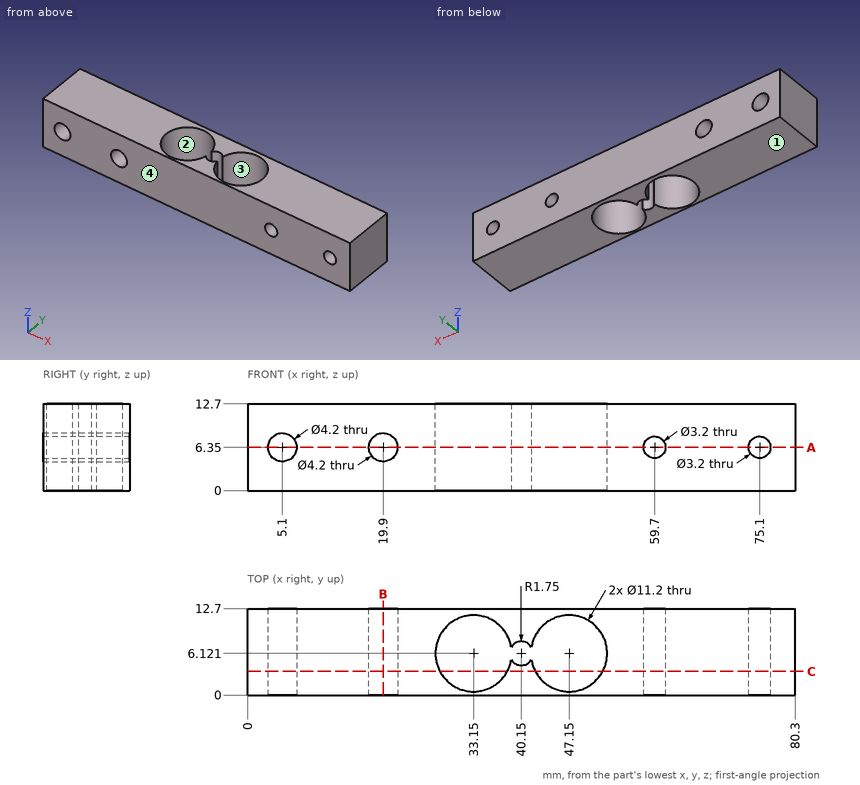
Study the drawing (mm; zero at the part's minimum x, y, z) and answer. Coordinates: 2 decimals unless noted, no trailing zeros. Order: outer loops, then holes, each group sorted by start corner. A loop starts at its lowest first (then second) coordinate and runs counter-clockwise, first axis right, second up. Notation, with made-up numbers: M 34.5,45.5 L 89.5,45.5 A28 cw 89.5,84.5 Z; hole C 48.25,45.5 d10. An arc over 180 degrees is marked long. Answer as a JSON object with one key per item and string values. Group by question number.
1. Straight lines are drawn through the part: line 1 (Y direction, x = 47.15, z = 6.75); line 2 (Z direction, x = 5.1, y = 6.75); line 3 (X direction, y = 6.25, z = 4). For each, find the intervals that lie inside material, in ascending order.
2. Section A-A on z = 6.35 is taken. State how many separate pieces and enclosed holes the cut face has, then the cut area to 3 significant figures.
3. Section C-C on y = 3.5 is taken. Write down the section's boundary in (x, z), then the cut area to 3 significant figures.
4. Section B-B on x = 19.9 is taken. Write down the section's boundary in (y, z).
5. A flat-ended cylindrical pin translates along its axis: P1, Ø2, axis at x = 43.5, y = 8, coming from the -Z side. Find the tip coordinate at first contact, or state that the pin passes through.
6. Determine the mould class of the marked faces 1, 2, 3 and 4 for opening direction Y: released by +Y, released by -Y, zero draft, split by the parting line, or undercut.
Values follow:
{
 "1": {"line 1": "0 to 0.52, 11.72 to 12.7", "line 2": "0 to 4.25, 8.45 to 12.7", "line 3": "0 to 27.55, 52.75 to 80.3"},
 "2": {"separate pieces": "5", "enclosed holes": "1", "area": "626 mm2"},
 "3": {"outline": "M 0,0 L 28.2,0 L 28.2,12.7 L 0,12.7 Z; M 38.1,0 L 42.2,0 L 42.2,12.7 L 38.1,12.7 Z; M 52.1,0 L 80.3,0 L 80.3,12.7 L 52.1,12.7 Z; hole C 5.1,6.35 d4.2; hole C 19.9,6.35 d4.2; hole C 59.7,6.35 d3.2; hole C 75.1,6.35 d3.2", "area": "725 mm2"},
 "4": {"outline": "M 0,0 L 12.7,0 L 12.7,4.25 L 0,4.25 Z; M 0,8.45 L 12.7,8.45 L 12.7,12.7 L 0,12.7 Z"},
 "5": {"P1": "through"},
 "6": {"face 1": "zero draft", "face 2": "undercut", "face 3": "undercut", "face 4": "released by -Y"}
}
